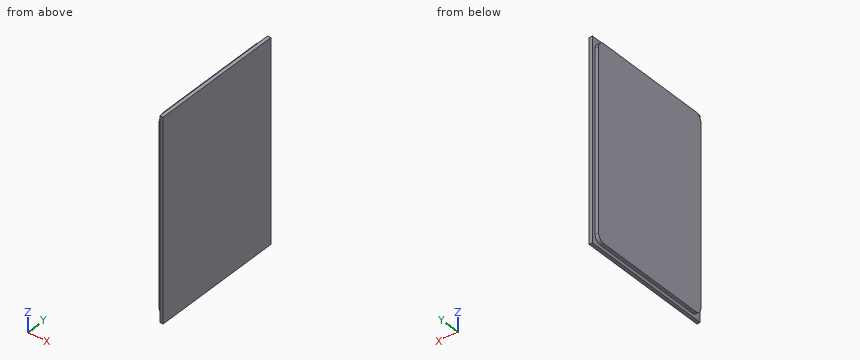
from build123d import *

# Parameters (mm, degrees)
SKETCH1_W           = 300
SKETCH1_H           = 200
BOSS_EXTRUDE1_DEPTH = 5
BOSS_EXTRUDE2_DEPTH = 5


with BuildPart() as part:
    # Sketch1 → Boss-Extrude1 (new body)
    with BuildSketch(Plane(origin=(0, 0, 0), x_dir=(0, 0, -1), z_dir=(1, 0, 0))):
        Rectangle(SKETCH1_W, SKETCH1_H)
    extrude(amount=BOSS_EXTRUDE1_DEPTH)

    # Sketch2 → Boss-Extrude2 (add)
    with BuildSketch(Plane.ZY):
        with BuildLine():
            Line((145, -85), (145, 85))
            ThreePointArc((145, 85), (142.071067812, 92.071067812), (135, 95))
            Line((135, 95), (-135, 95))
            ThreePointArc((-135, 95), (-142.071067812, 92.071067812), (-145, 85))
            Line((-145, 85), (-145, -85))
            ThreePointArc((-145, -85), (-142.071067812, -92.071067812), (-135, -95))
            Line((-135, -95), (135, -95))
            ThreePointArc((135, -95), (142.071067812, -92.071067812), (145, -85))
        make_face()
    extrude(amount=BOSS_EXTRUDE2_DEPTH)


solid = part.part
Verification items for the finished model (mm, model axes). Coordinates: 2 decimals unless noted, no trailing zeros. Order: outer loops, then holes, each group sorted by start corner. A loop starts at its lowest first (then second) coordinate and runs counter-clockwise, first axis right, second up. Notation, with made-up numbers: M -17.75,-1.5 L 7.25,-1.5 A28 cw 7.25,36.5 Z; hole C 15,88.25 d11. An arc over 180 degrees is marked long. One line per item, written item: value. Start each with the question number.
Item 1: Depth check by flat-ended pin: P1, Ø2, axis at x = -4, z = -12, coming from the +Y side; P2, Ø4, axis at x = -1.5, y = -6, coming from the +Z side. Enter the tip coordinate at first touch or a pass-through.
Item 2: Sectioned sample at B-B on z = -33. Record the cut outline in (x, y).
Item 3: Thickness scan on probe 1 along Y at (x, z) = (-1.75, 62.5); probe 2 along Z at (x, y) = (-3, -3). Record the ranges inside material, lowest first.
Item 4: Sectioned sample at A-A on x = -2.5. Record the cut outline in (y, z), then the cut area to 3 significant figures.
Calculated:
1. P1: y = 95
1. P2: z = 150
2. outline: M -5,-95 L 0,-95 L 0,-100 L 5,-100 L 5,100 L 0,100 L 0,95 L -5,95 Z
3. probe 1: -95 to 95
3. probe 2: -145 to 145
4. outline: M -95,-135 A10 ccw -85,-145 L 85,-145 A10 ccw 95,-135 L 95,135 A10 ccw 85,145 L -85,145 A10 ccw -95,135 Z
4. area: 55,000 mm^2
